Build history of the part. All positions in model axes, mm. Round coordinates to 2 decimals unless told otherwise and drop trailing zeros. Order: outer loops, then holes, each group sorted by start corner. A loop starts at its lowest first (then second) coordinate and runs counter-clockwise, first axis right, second up. Notation, with made-up numbers: (-20.5, 42) -> (33.5, 42) arc R14 ccw to (33.5, 47) -> close; hole circle Ø2 at (12, 54.5). An arc over 180 degrees is marked (long way). Answer as a JSON object with one key per item and string values.
Autodesk Inventor part; units mm, degrees
ref_plane "YZ Plane" through (0, 0, 0) normal (1, 0, 0) x (0, 1, 0)
ref_plane "XZ Plane" through (0, 0, 0) normal (0, 1, 0) x (-1, 0, 0)
ref_plane "XY Plane" through (0, 0, 0) normal (0, 0, 1) x (1, 0, 0)
sketch "Sketch1" plane through (0, 0, 0) normal (0, 0, 1) x (1, 0, 0)
  line L0 (45, -50) -> (-45, -50)
  line L1 (-45, -50) -> (-45, 50)
  line L2 (-45, 50) -> (45, 50)
  line L3 (45, 50) -> (45, -50)
  line L4 (45, -50) -> (-45, 50) construction
  line L5 (-45, -50) -> (45, 50) construction
  line L6 (53, 58) -> (-53, 58)
  line L7 (-53, 58) -> (-53, 54.5)
  line L8 (-53, -58) -> (53, -58)
  line L9 (53, -58) -> (53, -54.5)
  line L10 (-20, 50) -> (20, 50)
  line L11 (20, 50) -> (20, 54)
  line L12 (20, 54) -> (-20, 54)
  line L13 (-20, 54) -> (-20, 50)
  line L14 (-20, -50) -> (20, -50)
  line L15 (20, -50) -> (20, -54)
  line L16 (20, -54) -> (-20, -54)
  line L17 (-20, -54) -> (-20, -50)
  line L18 (-45, 20) -> (-49, 20)
  line L19 (-49, 20) -> (-49, -20)
  line L20 (-49, -20) -> (-45, -20)
  line L21 (-45, -20) -> (-45, 20)
  line L22 (45, 20) -> (49, 20)
  line L23 (49, 20) -> (49, -20)
  line L24 (49, -20) -> (45, -20)
  line L25 (45, -20) -> (45, 20)
  line L26 (-53, 6.5) -> (-77, 6.5)
  line L27 (-100, 6.5) -> (-100, -6.5)
  line L28 (-100, -6.5) -> (-92, -6.5)
  line L29 (-53, -6.5) -> (-53, 6.5) construction
  line L30 (-53, 0) -> (53, 0)
  circle A0 centre (-92, 0) radius 2.55
  circle A1 centre (-77, 0) radius 2.55
  line L31 (0, 50) -> (0, -50)
  line L32 (-53, 6.5) -> (-53, -6.5) construction
  line L33 (-53, -6.5) -> (-53, -44.5)
  line L34 (53, 6.5) -> (53, 44.5)
  line L35 (53, -6.5) -> (53, 6.5) construction
  line L36 (-92, -6.5) -> (-77, -6.5) construction
  line L37 (-77, -6.5) -> (-77, -44.5)
  line L38 (-77, -58) -> (-92, -58) construction
  line L39 (-92, -58) -> (-92, -54.5) construction
  line L40 (-92, -58) -> (-77, -58) construction
  line L41 (-77, -58) -> (-77, -58.5) construction
  line L42 (-77, -58.5) -> (-81.5, -58.5) construction
  line L43 (-92, -58.5) -> (-92, -58) construction
  line L44 (-92, -54.5) -> (-87.5, -54.5)
  line L45 (-87.5, -54.5) -> (-87.5, -58.5)
  line L46 (-81.5, -58.5) -> (-81.5, -54.5)
  line L47 (-81.5, -54.5) -> (-77, -54.5)
  line L48 (-77, 6.5) -> (-77, 44.5)
  line L49 (-77, 58) -> (-92, 58) construction
  line L50 (-92, 58) -> (-92, 54.5) construction
  line L51 (-92, 58) -> (-77, 58) construction
  line L52 (-77, 58) -> (-77, 58.5) construction
  line L53 (-77, 58.5) -> (-81.5, 58.5) construction
  line L54 (-92, 58.5) -> (-92, 58) construction
  line L55 (-92, 54.5) -> (-87.5, 54.5)
  line L56 (-87.5, 54.5) -> (-87.5, 58.5)
  line L57 (-81.5, 58.5) -> (-81.5, 54.5)
  line L58 (-81.5, 54.5) -> (-77, 54.5)
  line L59 (-77, 6.5) -> (-92, 6.5) construction
  line L60 (-92, 6.5) -> (-100, 6.5)
  line L61 (-92, -6.5) -> (-77, -6.5) construction
  line L62 (-77, -6.5) -> (-53, -6.5)
  line L63 (-77, 54.5) -> (-77, 58) construction
  line L64 (-92, 54.5) -> (-92, 6.5)
  line L65 (-87.5, 58.5) -> (-92, 58.5) construction
  line L66 (-81.5, 58.5) -> (-87.5, 58.5)
  line L67 (-92, -54.5) -> (-92, -6.5)
  line L68 (-87.5, -58.5) -> (-92, -58.5) construction
  line L69 (-81.5, -58.5) -> (-87.5, -58.5)
  line L70 (-77, -54.5) -> (-77, -58) construction
  line L71 (-77, 54.5) -> (-71.5, 54.5)
  line L72 (-53, 54.5) -> (-53, 44.5) construction
  line L73 (-53, 44.5) -> (-77, 44.5)
  line L74 (-77, 44.5) -> (-77, 54.5) construction
  line L75 (-77, -54.5) -> (-71.5, -54.5)
  line L76 (-53, -54.5) -> (-53, -54)
  line L77 (-53, -44.5) -> (-77, -44.5)
  line L78 (-77, -44.5) -> (-77, -54.5) construction
  line L79 (-71.5, 54.5) -> (-65.5, 54.5) construction
  line L80 (-65.5, 54.5) -> (-65.5, 58.5)
  line L81 (-65.5, 58.5) -> (-71.5, 58.5)
  line L82 (-71.5, 58.5) -> (-71.5, 54.5)
  line L83 (-71.5, -54.5) -> (-65.5, -54.5) construction
  line L84 (-65.5, -54.5) -> (-65.5, -58.5)
  line L85 (-65.5, -58.5) -> (-71.5, -58.5)
  line L86 (-71.5, -58.5) -> (-71.5, -54.5)
  line L87 (-71.5, 54.5) -> (-65.5, 54.5) construction
  line L88 (-65.5, 54.5) -> (-53, 54.5)
  line L89 (-77, 44.5) -> (-77, 54.5) construction
  line L90 (-53, 44.5) -> (-53, 6.5)
  line L91 (-53, 54.5) -> (-53, 44.5) construction
  line L92 (-77, -44.5) -> (-77, -54.5) construction
  line L93 (-53, -44.5) -> (-53, -54.5) construction
  line L94 (-53, -54) -> (-53, -44.5) construction
  line L95 (-65.5, -54.5) -> (-53, -54.5)
  line L96 (-71.5, -54.5) -> (-65.5, -54.5) construction
  line L97 (-53, -54.5) -> (-53, -58)
  line L98 (53, 6.5) -> (77, 6.5)
  line L99 (100, 6.5) -> (100, -6.5)
  line L100 (100, -6.5) -> (92, -6.5)
  circle A2 centre (92, 0) radius 2.55
  circle A3 centre (77, 0) radius 2.55
  line L101 (92, -6.5) -> (77, -6.5) construction
  line L102 (77, -6.5) -> (77, -44.5)
  line L103 (77, -58) -> (92, -58) construction
  line L104 (92, -58) -> (92, -54.5) construction
  line L105 (92, -58) -> (77, -58) construction
  line L106 (77, -58) -> (77, -58.5) construction
  line L107 (77, -58.5) -> (81.5, -58.5) construction
  line L108 (92, -58.5) -> (92, -58) construction
  line L109 (92, -54.5) -> (87.5, -54.5)
  line L110 (87.5, -54.5) -> (87.5, -58.5)
  line L111 (81.5, -58.5) -> (81.5, -54.5)
  line L112 (81.5, -54.5) -> (77, -54.5)
  line L113 (92, 54.5) -> (87.5, 54.5)
  line L114 (92, 58) -> (92, 54.5) construction
  line L115 (77, 6.5) -> (77, 44.5)
  line L116 (81.5, 54.5) -> (77, 54.5)
  line L117 (77, 58) -> (92, 58) construction
  line L118 (92, 58) -> (77, 58) construction
  line L119 (77, 58) -> (77, 58.5) construction
  line L120 (77, 58.5) -> (81.5, 58.5) construction
  line L121 (81.5, 58.5) -> (81.5, 54.5)
  line L122 (92, 58.5) -> (92, 58) construction
  line L123 (87.5, 54.5) -> (87.5, 58.5)
  line L124 (77, 6.5) -> (92, 6.5) construction
  line L125 (92, 6.5) -> (100, 6.5)
  line L126 (92, -6.5) -> (77, -6.5) construction
  line L127 (77, -6.5) -> (53, -6.5)
  line L128 (77, 54.5) -> (77, 58) construction
  line L129 (92, 54.5) -> (92, 6.5)
  line L130 (87.5, 58.5) -> (92, 58.5) construction
  line L131 (81.5, 58.5) -> (87.5, 58.5)
  line L132 (92, -54.5) -> (92, -6.5)
  line L133 (87.5, -58.5) -> (92, -58.5) construction
  line L134 (81.5, -58.5) -> (87.5, -58.5)
  line L135 (77, -54.5) -> (77, -58) construction
  line L136 (77, 54.5) -> (71.5, 54.5)
  line L137 (53, 44.5) -> (77, 44.5)
  line L138 (77, 44.5) -> (77, 54.5) construction
  line L139 (77, -54.5) -> (71.5, -54.5)
  line L140 (53, -44.5) -> (77, -44.5)
  line L141 (77, -44.5) -> (77, -54.5) construction
  line L142 (71.5, 54.5) -> (65.5, 54.5) construction
  line L143 (65.5, 54.5) -> (65.5, 58.5)
  line L144 (65.5, 58.5) -> (71.5, 58.5)
  line L145 (71.5, 58.5) -> (71.5, 54.5)
  line L146 (71.5, -54.5) -> (65.5, -54.5) construction
  line L147 (65.5, -54.5) -> (65.5, -58.5)
  line L148 (65.5, -58.5) -> (71.5, -58.5)
  line L149 (71.5, -58.5) -> (71.5, -54.5)
  line L150 (71.5, 54.5) -> (65.5, 54.5) construction
  line L151 (65.5, 54.5) -> (53, 54.5)
  line L152 (77, 44.5) -> (77, 54.5) construction
  line L153 (77, -44.5) -> (77, -54.5) construction
  line L154 (65.5, -54.5) -> (53, -54.5)
  line L155 (71.5, -54.5) -> (65.5, -54.5) construction
  line L156 (53, 44.5) -> (53, 54.5) construction
  line L157 (53, 54.5) -> (53, 58)
  line L158 (53, -44.5) -> (53, -6.5)
  line L159 (53, -54.5) -> (53, -44.5) construction
  point P0 (0, 0)
  point P1 (0, 54)
  point P2 (0, 0)
  point P3 (-49, 0)
  point P4 (0, 0)
  point P5 (-53, 0)
  point P6 (0, 0)
  point P7 (0, 0)
  point P8 (-84.5, -58)
  point P9 (-84.5, 58)
  point P10 (-65, 44.5)
  point P11 (-81.5, 56.5)
  point P12 (-71.5, 56.5)
  point P13 (84.5, -58)
  point P14 (84.5, 58)
  point P15 (65, 44.5)
  point P16 (81.5, 56.5)
  point P17 (71.5, 56.5)
  dimension "d0" = 100
  dimension "d1" = 90
  dimension "d2" = 8
  dimension "d3" = 4
  dimension "d4" = 4
  dimension "d5" = 40
  dimension "d6" = 40
  dimension "d7" = 4
  dimension "d8" = 4
  dimension "d9" = 13
  dimension "d10" = 47
  dimension "d11" = 5.1
  dimension "d12" = 15
  dimension "d13" = 24
  dimension "d14" = 4
  dimension "d15" = 4
  dimension "d16" = 15
  dimension "d17" = 0.5
  dimension "d18" = 6
  dimension "d19" = 4.5
  dimension "d20" = 4.5
  dimension "d21" = 4
  dimension "d24" = 10
  dimension "d25" = 10
  dimension "d27" = 10
  dimension "d28" = 6
extrude "Extrusion1" add sketch "Sketch1" along normal blind 4
properties part number "DoorFrameRearL2_V3" material "Wood (Oak)"
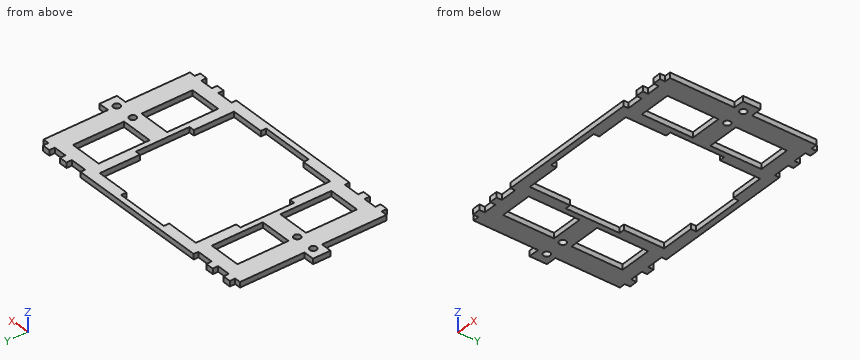
1) Cut at B-B, the plane y = -12. Give the cut face in (x, z).
Checked values:
{"outline": "(-92, 0) -> (-77, 0) -> (-77, 4) -> (-92, 4) -> close; (-53, 0) -> (-49, 0) -> (-49, 4) -> (-53, 4) -> close; (49, 0) -> (53, 0) -> (53, 4) -> (49, 4) -> close; (77, 0) -> (92, 0) -> (92, 4) -> (77, 4) -> close"}
2) Cut at D-D, the plane z = 2.6. Count the separate pieces of the cut face and the enclosed holes in it, plus the area to 3 significant figures.
Checked values:
{"separate pieces": "1", "enclosed holes": "9", "area": "7,830 mm²"}
3) Cut at C-C, the plane y = 0. Give the cut face in (x, z).
Checked values:
{"outline": "(-100, 0) -> (-94.55, 0) -> (-94.55, 4) -> (-100, 4) -> close; (-89.45, 0) -> (-79.55, 0) -> (-79.55, 4) -> (-89.45, 4) -> close; (-74.45, 0) -> (-49, 0) -> (-49, 4) -> (-74.45, 4) -> close; (49, 0) -> (74.45, 0) -> (74.45, 4) -> (49, 4) -> close; (79.55, 0) -> (89.45, 0) -> (89.45, 4) -> (79.55, 4) -> close; (94.55, 0) -> (100, 0) -> (100, 4) -> (94.55, 4) -> close"}
4) Probe L1, parallel to X at y = -19, z = 2.65; L2, parallel to X at y = 29.5, z = 3.25; L3, parallel to Y at x = -56, z = 0.8. List the from-to ranges inside material, lowest first. Write a range as from..to.
Checked values:
{"L1": "x = -92..-77, -53..-49, 49..53, 77..92", "L2": "x = -92..-77, -53..-45, 45..53, 77..92", "L3": "y = -54.5..-44.5, -6.5..6.5, 44.5..54.5"}
5) Cut at A-A, the plane x = 16. Give the cut face in (y, z), plus the area to 3 significant figures.
Checked values:
{"outline": "(-58, 0) -> (-54, 0) -> (-54, 4) -> (-58, 4) -> close; (54, 0) -> (58, 0) -> (58, 4) -> (54, 4) -> close", "area": "32.0 mm²"}
6) Flat gauge pins, fed straight in: pin 1 Ø1 at (y, z) = (-56, 3) entering from +X; pin 2 Ø2 at (y, z) = (52.5, 2.5) entering from +X; pin 3 Ø3 at (x, y) = (92, 0) entering from -Z; pin 4 Ø2 at (x, z) = (-1.5, 2.5) entering from -Y. Where does each tip first touch, or does it go through?
Checked values:
{"pin 1": "stops at x = 87.5", "pin 2": "stops at x = 92", "pin 3": "passes through", "pin 4": "stops at y = -58"}
